Geometry: final body of the model. Coordinates: model frame, mm. Round coordinates to 2 decimals unless told otherwise and drop trailing zeros. Loops run counter-clockwise (first coordinate to the right, second up) from the corner with the lowest first, then second, coordinate; pieces in that order, holes last. Notation, with made-up numbers: (28.25, 32) -> (48.25, 32) arc R16 cw to (48.25, 60) -> close; hole circle Ø5 at (66, 44). An arc over 180 degrees is marked (long way). Answer in a Markdown table with one row per item.
Autodesk Inventor part; units mm, degrees
ref_plane "YZ Plane" through (0, 0, 0) normal (1, 0, 0) x (0, 1, 0)
ref_plane "XZ Plane" through (0, 0, 0) normal (0, 1, 0) x (-1, 0, 0)
ref_plane "XY Plane" through (0, 0, 0) normal (0, 0, 1) x (1, 0, 0)
sketch "Sketch1" plane through (0, 0, 0) normal (0, 0, 1) x (1, 0, 0)
  line L0 (0, 0) -> (207, 0)
  line L1 (207, 0) -> (207, 40)
  line L2 (207, 40) -> (0, 40)
  line L3 (0, 40) -> (0, 0)
  dimension "d0" = 207
  dimension "d1" = 40
extrude "Extrusion1" add sketch "Sketch1" along normal blind 5
sketch "Sketch2" plane through (0, 0, 5) normal (0, 0, 1) x (1, 0, 0)
  line L0 (207, 40) -> (0, 40)
  line L1 (0, 0) -> (207, 0)
  line L2 (0, 40) -> (0, 0)
  point P0 (17.5, 32.5)
  point P1 (17.5, 7.5)
  point P2 (112.5, 32.5)
  point P3 (112.5, 7.5)
  point P4 (186.5, 32.5)
  point P5 (186.5, 7.5)
  dimension "d4" = 7.5
  dimension "d5" = 7.5
  dimension "d6" = 17.5
  dimension "d7" = 95
  dimension "d8" = 74
hole "Hole1" at (17.5, 32.5, 5) at (17.5, 7.5, 5) at (112.5, 32.5, 5) at (112.5, 7.5, 5) at (186.5, 32.5, 5) at (186.5, 7.5, 5) direction (0, 0, -1) diameter 4.5 end through all countersink diameter 9.4 countersink angle 90
sketch "Sketch3" plane through (0, 0, 5) normal (0, 0, 1) x (1, 0, 0)
  line L0 (0, 40) -> (0, 0)
  line L1 (0, 0) -> (207, 0)
  circle A0 centre (186.5, 7.5) radius 4.7
  point P0 (159, 32)
  dimension "d17" = 32
  dimension "d25" = 27.5
hole "Hole2" [suppressed]
sketch "Sketch4" plane through (0, 0, 5) normal (0, 0, 1) x (1, 0, 0)
  line L0 (207, 40) -> (0, 40)
  line L1 (0, 40) -> (0, 0)
  point P0 (40, 30)
  point P1 (140, 30)
  dimension "d26" = 100
  dimension "d27" = 10
  dimension "d28" = 40
hole "Hole3" at (40, 30, 5) at (140, 30, 5) direction (0, 0, -1) diameter 3.4 end through all
properties part number "Top_Slider Piece 3" material "Wood (Oak)"
Item 1: Section query C-C, the plane x = 40. Output: boundary loops of the cut face in (y, z).
Ans:
| item | result |
|---|---|
| outline | (0, 0) -> (28.3, 0) -> (28.3, 5) -> (0, 5) -> close; (31.7, 0) -> (40, 0) -> (40, 5) -> (31.7, 5) -> close |
Item 2: Mould query, pull axis Y, two halves, no side actions, for faces 1 (the conical face through (184.154, 33.021, 2.703)), 2 (the flat face through (102, 20, 5)), 3 (the flat face through (102, 0, 2)), 4 (the flat face through (105, 40, 2)). Classes: released by +Y, released by -Y, zero draft, split by the parting line, or undercut.
Ans:
| item | result |
|---|---|
| face 1 | undercut |
| face 2 | zero draft |
| face 3 | released by -Y |
| face 4 | released by +Y |
Item 3: Section query A-A, the plane x = 186.5. Output: boundary loops of the cut face in (y, z), and give its area (3 significant figures).
Ans:
| item | result |
|---|---|
| outline | (0, 0) -> (5.25, 0) -> (5.25, 2.55) -> (2.8, 5) -> (0, 5) -> close; (9.75, 0) -> (30.25, 0) -> (30.25, 2.55) -> (27.8, 5) -> (12.2, 5) -> (9.75, 2.55) -> close; (34.75, 0) -> (40, 0) -> (40, 5) -> (37.2, 5) -> (34.75, 2.55) -> close |
| area | 143 mm2 |
Item 4: Ray query, L1, parallel to X at y = 7.5, z = 1.25; L2, parallel to Y at x = 17.5, z = 1.6; L3, parallel to X at y = 30, z = 0.6. Return the intervals inside material, ascending.
Ans:
| item | result |
|---|---|
| L1 | 0 to 15.25, 19.75 to 110.25, 114.75 to 184.25, 188.75 to 207 |
| L2 | 0 to 5.25, 9.75 to 30.25, 34.75 to 40 |
| L3 | 0 to 38.3, 41.7 to 138.3, 141.7 to 207 |
Item 5: Section query B-B, the plane z = 3.3. State how many separate pieces and enclosed holes the cut face has, and give its area (3 significant figures).
Ans:
| item | result |
|---|---|
| separate pieces | 1 |
| enclosed holes | 8 |
| area | 8,090 mm2 |
Item 6: First-contact query: P1, Ø2.5, axis at x = 112.5, y = 7.5, coming from the +Z side; P2, Ø5, axis at x = 186.5, y = 32.5, coming from the +Z side. Flat tips, straight axial feed; report the tip coordinate or a pass-through.
Ans:
| item | result |
|---|---|
| P1 | through |
| P2 | z = 2.8 |
